For this review, take the finished solid that the model builds, in its own axes (mm). Give positions to 0.01 mm unless a question says otherwise; leave off trailing zeros. Write each loop counter-clockwise with the first axis right and the second up, starting at its lowest first coordinate (ties: lowest second). Pieces come first, ordered by that corner, then holes.
1) For P1, Ø6, axis at y = -14.5, z = 56, coming from the -X side; P2, Ø6, axis at x = -192.5, y = -11.5, coming from the -Z side; P3, Ø6, axis at y = -10.5, z = 70, coming from the +X side; P4, Ø4, axis at x = 58, z = 1, coming from the +Y side, all flat-tipped, find the tip position at first contact; note any pin that passes through.
2) We need section A-A on z = 64. Give the boundary of the cut face in (x, y).
3) Wall thickness on line 1 along X through (y, z) = (-8.75, 13); line 2 along X through (y, z) = (-10.25, 52): over which ranges is each line inside the solid? List them lowest first.
4) We need section C-C on z = 15. Give the boundary of the cut face in (x, y).
5) We need section B-B on y = -12.75. Give the boundary of the cut face in (x, z), and give its area (3 significant figures).
from build123d import *

# Parameters (mm, degrees)
F0_W     = 20
F0_H     = 18.615236
F0_H_2   = 18.615237
F1_DEPTH = 20
F3_DEPTH = 20


with BuildPart() as f1:
    # F0 (on Front) → F1 (new body)
    with BuildSketch(Plane.XZ):
        Polygon((-179.463843, 107.230473), (-199.463843, 107.230473), (-199.463843, 74.172214), (-179.463843, 74.172214), (-179.463843, 37.230473), (-179.463843, 18.615237), (-179.463843, 0), (-179.463843, -32.769527), (140.536157, -32.769527), (140.536157, 107.230473), align=None)
        with Locations((-189.463843, 27.922855)):
            Rectangle(F0_W, F0_H)
        with Locations((-189.463843, 9.307619)):
            Rectangle(F0_W, F0_H_2)
    extrude(amount=F1_DEPTH)

    # F2 (on face) → F3 (cut)
    with BuildSketch(Plane.YZ.offset(140.536157)):
        Polygon((-20, 84.144631), (-20, 55.335836), (0, 46.306214), (0, 93.604238), align=None)
        Polygon((0, 28.154733), (-20, 19.125111), (-20, -9.683684), (0, -19.143291), align=None)
    extrude(amount=-F3_DEPTH, mode=Mode.SUBTRACT)


solid = f1.part
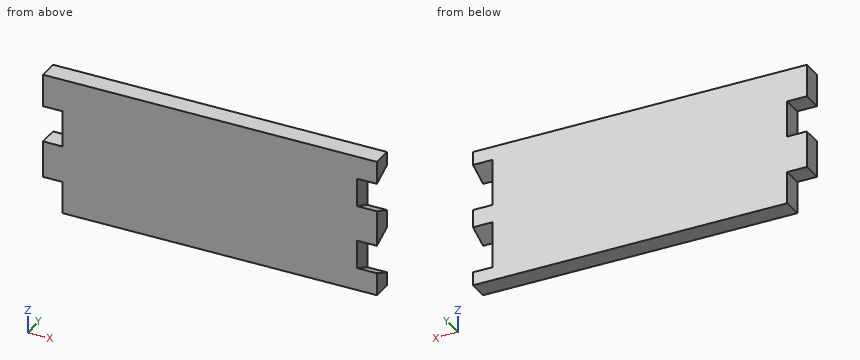
Results list:
1. P1: stops at x = -179.46
1. P2: stops at z = 0
1. P3: stops at x = 120.54
1. P4: stops at y = 0
2. outline: (-179.46, -20) - (120.54, -20) - (120.54, 0) - (-179.46, 0) - close
3. line 1: x = -199.46 to 120.54
3. line 2: x = -179.46 to 120.54
4. outline: (-199.46, -20) - (120.54, -20) - (120.54, 0) - (-199.46, 0) - close
5. outline: (-199.46, 0) - (-179.46, 0) - (-179.46, -32.77) - (140.54, -32.77) - (140.54, -13.11) - (120.54, -13.11) - (120.54, 22.4) - (140.54, 22.4) - (140.54, 52.06) - (120.54, 52.06) - (120.54, 87.57) - (140.54, 87.57) - (140.54, 107.23) - (-199.46, 107.23) - (-199.46, 74.17) - (-179.46, 74.17) - (-179.46, 37.23) - (-199.46, 37.23) - close
5. area: 44,800 mm2
